Read the model definition and answer for the solid it produces. Units are mm, in the model's axes. Face numbers are marked on the shaded views. A direction names the side the tool comes from. Give positions to 0.01 mm unless a question says otherwise; leave off trailing zeros. Order: outer loops, then holes, each group sorted by start corner. A loop starts at its lowest first (then second) coordinate and runs counter-clockwise, first axis right, second up. Notation, with made-up numbers: (43.5, 23.25) - (100.5, 23.25) arc R11 cw to (100.5, 34.25) - close; hole circle Ø5 at (-11, 28). An arc over 180 degrees is marked (long way). Return JSON: item names as keys, results as strings.
```python
from build123d import *

# Parameters (mm, degrees)
SKETCH1_W              = 109.474
SKETCH1_H              = 76.962
BOSS_EXTRUDE1_DEPTH    = 1.016
SKETCH2_W              = 109.474
SKETCH2_H              = 1.016
BOSS_EXTRUDE2_DEPTH    = 36.322
SKETCH3_R              = 1.6383
CUT_EXTRUDE1_DEPTH     = 139.661435893
SKETCH4_W              = 86.36
SKETCH4_H              = 75.946
BOSS_EXTRUDE3_DEPTH    = 36.322
SKETCH5_R              = 1.6383
SKETCH5_R_2            = 1.143
CUT_EXTRUDE2_DEPTH     = 1.016
SKETCH6_R              = 1.143
CUT_EXTRUDE3_DEPTH     = 6.35
SKETCH7_W              = 1.524
SKETCH7_H              = 75.946
BOSS_EXTRUDE4_DEPTH    = 15.24
CUT_EXTRUDE4_REACH     = 139.08
SKETCH8_W              = 7.62
SKETCH8_H              = 6.858
SKETCH9_W              = 15.24
SKETCH9_H              = 48.768
BOSS_EXTRUDE5_DEPTH    = 8.128
SKETCH10_R             = 2.794
BOSS_EXTRUDE6_DEPTH    = 3.81
FILLET1_R              = 1.5875
LPATTERN2_COUNT        = 5
LPATTERN2_PITCH        = 9.144
FILLET1_OF_LPATTERN2_R = 1.5875
BOSS_EXTRUDE7_DEPTH    = 65.786


with BuildPart() as part:
    # Sketch1 → Boss-Extrude1 (new body)
    with BuildSketch(Plane.XY):
        with Locations((54.737, 38.481)):
            Rectangle(SKETCH1_W, SKETCH1_H)
    extrude(amount=BOSS_EXTRUDE1_DEPTH)

    # Sketch2 → Boss-Extrude2 (add)
    with BuildSketch(Plane.XY.offset(1.016)):
        with Locations((54.737, 76.454)):
            Rectangle(SKETCH2_W, SKETCH2_H)
    extrude(amount=BOSS_EXTRUDE2_DEPTH)

    # Sketch3 → Cut-Extrude1 (cut, through all)
    with BuildSketch(Plane.XY.offset(1.016)):
        with Locations((104.6861, 71.2343)):
            Circle(SKETCH3_R)
        with BuildLine():
            Line((2.2225, 2.286), (0, 2.286))
            Line((0, 2.286), (0, 5.969))
            Line((0, 5.969), (2.2225, 5.969))
            ThreePointArc((2.2225, 5.969), (4.064, 4.1275), (2.2225, 2.286))
        make_face()
    extrude(amount=-CUT_EXTRUDE1_DEPTH, mode=Mode.SUBTRACT)

    # Sketch4 → Boss-Extrude3 (add)
    with BuildSketch(Plane.XY.offset(1.016)):
        with Locations((51.054, 37.973)):
            Rectangle(SKETCH4_W, SKETCH4_H)
    extrude(amount=BOSS_EXTRUDE3_DEPTH)

    # Sketch5 → Cut-Extrude2 (cut)
    with BuildSketch(Plane(origin=(0, 76.962, 0), x_dir=(1, 0, 0), z_dir=(0, 1, 0))):
        with Locations(Location((104.5337, -28.5877, 0), (0, 0, 270))):
            Circle(SKETCH5_R)
        with Locations(Location((99.5426, -19.177, 0), (0, 0, 270))):
            Circle(SKETCH5_R_2)
        with Locations(Location((12.065, -13.208, 0), (0, 0, 270))):
            Circle(SKETCH5_R_2)
        with BuildLine():
            Line((2.9337, -26.9494), (0, -26.9494))
            Line((0, -26.9494), (0, -30.226))
            Line((0, -30.226), (2.9337, -30.226))
            ThreePointArc((2.9337, -30.226), (4.572, -28.5877), (2.9337, -26.9494))
        make_face()
    extrude(amount=-CUT_EXTRUDE2_DEPTH, mode=Mode.SUBTRACT)

    # Sketch6 → Cut-Extrude3 (cut)
    with BuildSketch(Plane(origin=(0, 0, 0), x_dir=(-1, 0, 0), z_dir=(0, 0, -1))):
        with Locations((-78.1304, 24.8412)):
            Circle(SKETCH6_R)
        with Locations((-42.3164, 24.8412)):
            Circle(SKETCH6_R)
        with Locations((-42.3164, 52.5272)):
            Circle(SKETCH6_R)
    extrude(amount=-CUT_EXTRUDE3_DEPTH, mode=Mode.SUBTRACT)

    # Sketch7 → Boss-Extrude4 (add)
    with BuildSketch(Plane(origin=(94.234, 0, 0), x_dir=(0, 0, -1), z_dir=(1, 0, 0))):
        with Locations((-6.858, 37.973)):
            Rectangle(SKETCH7_W, SKETCH7_H)
    extrude(amount=BOSS_EXTRUDE4_DEPTH)

    # Sketch8 → Cut-Extrude4 (cut, up to next)
    with BuildSketch(Plane.XY.offset(7.62), mode=Mode.PRIVATE) as cut_extrude4_sk1:
        with Locations((105.664, 72.517)):
            Rectangle(SKETCH8_W, SKETCH8_H)
    cut_extrude4_tool1 = extrude(cut_extrude4_sk1.sketch, amount=-CUT_EXTRUDE4_REACH, mode=Mode.PRIVATE) & part.part
    add(cut_extrude4_tool1.solids().sort_by_distance((105.664, 72.517, 7.62))[0], mode=Mode.SUBTRACT)

    # Sketch9 → Boss-Extrude5 (add)
    with BuildSketch(Plane.XY.offset(7.62)):
        with Locations((101.854, 34.544)):
            Rectangle(SKETCH9_W, SKETCH9_H)
    extrude(amount=BOSS_EXTRUDE5_DEPTH)

    # Sketch10 → Boss-Extrude6 (add)
    with BuildSketch(Plane.XY.offset(15.748)):
        with Locations(Location((103.886, 15.748, 0), (0, 0, 180))):
            Circle(SKETCH10_R)
    boss_extrude6 = extrude(amount=BOSS_EXTRUDE6_DEPTH)

    # Fillet1
    fillet1_edges = [part.edges().sort_by_distance(p)[0] for p in [
        (106.68, 15.748, 19.558),
    ]]
    fillet(fillet1_edges, radius=FILLET1_R)

    # LPattern2: Boss-Extrude6 ×5
    with Locations(*[(0, i * LPATTERN2_PITCH, 0) for i in range(1, LPATTERN2_COUNT)]):
        add(boss_extrude6)

    # Fillet1 of LPattern2
    fillet1_of_lpattern2_edges = [part.edges().sort_by_distance(p)[0] for p in [
        (106.68, 24.892, 19.558),
        (106.68, 34.036, 19.558),
        (106.68, 43.18, 19.558),
        (106.68, 52.324, 19.558),
    ]]
    fillet(fillet1_of_lpattern2_edges, radius=FILLET1_OF_LPATTERN2_R)

    # Sketch11 → Boss-Extrude7 (add)
    with BuildSketch(Plane.XZ.offset(-75.946)):
        Polygon((7.874, 1.016), (0, 1.016), (0, 6.096), (7.874, 11.176), align=None)
    extrude(amount=BOSS_EXTRUDE7_DEPTH)


solid = part.part
```
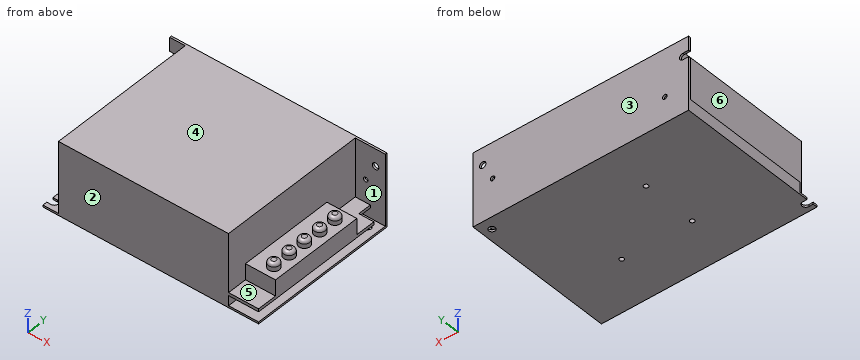
Q1. Consider L1, parallel to Z at x = 103.5, y = 56; L2, parallel to Y at x = 6, z = 19; L3, parallel to X at y = 38, z = 25. Determine where each line is inside the solid, lowest interval first.
Values:
{"L1": "z = 0 to 1.02, 6.1 to 15.75", "L2": "y = 75.95 to 76.96", "L3": "x = 7.87 to 94.23"}
Q2. For the marked faces 4, 5 and 6, determine the directions among +Z, -Z, +X, -X, +Y, -Y from which every point of the face is accessible in a straight line to the end or side of a thin tool.
Values:
{"face 4": "+Z, +X, -X, +Y, -Y", "face 5": "+Z, +X, -Y", "face 6": "+Z, -X, -Y"}
Q3. Given pin 1 (0.7 mm diameter, centred on x = 103.5, y = 24.5, fed in from +Z); pin 2 (4.5 mm diameter, centred on x = 102, z = 22, fed in from -Y), each flat-ended and moving along its own axis, determine where each tip first touches the part or whether it passes through.
Values:
{"pin 1": "stops at z = 19.56", "pin 2": "stops at y = 75.95"}
Q4. A cutting plane is placed at B-B (z = 3). Write down the section's boundary in (x, y).
Values:
{"outline": "(0, 10.16) - (7.87, 10.16) - (7.87, 0) - (94.23, 0) - (94.23, 75.95) - (109.47, 75.95) - (109.47, 76.96) - (0, 76.96) - close; hole circle Ø2.29 at (42.32, 24.84); hole circle Ø2.29 at (42.32, 52.53); hole circle Ø2.29 at (78.13, 24.84)"}
Q5. Determine the mould class of the marked faces 1, 2 and 3 for opening direction Y: released by +Y, released by -Y, zero draft, split by the parting line, or undercut.
Values:
{"face 1": "undercut", "face 2": "released by -Y", "face 3": "released by +Y"}
Q6. A cutting plane is placed at A-A (z = 28.5). Write down the section's boundary in (x, y), and give its area (3 significant figures).
Values:
{"outline": "(4.57, 75.95) - (7.87, 75.95) - (7.87, 0) - (94.23, 0) - (94.23, 75.95) - (102.9, 75.95) - (102.9, 76.96) - (4.57, 76.96) - close; (106.17, 75.95) - (109.47, 75.95) - (109.47, 76.96) - (106.17, 76.96) - close", "area": "6,660 mm²"}
